CAD build for the part. Positions are in the model's coordinates, mm. Coordinates: 2 decimals unless noted, no trailing zeros. Write each loop counter-clockwise with the first axis right and the second up, starting at its lowest first coordinate (ties: lowest second). Pieces come first, ordered by that corner, then holes. Notation, with made-up numbers: (81.25, 11) -> (102.25, 11) arc R26 ccw to (102.25, 39) -> close; hole circle Ø1 at (46.5, 55.25). An arc over 180 degrees is marked (long way). Answer as CSV lines item,"result".
```python
from build123d import *

# Parameters (mm, degrees)
SKETCH1_W           = 10
SKETCH1_H           = 5
BOSS_EXTRUDE1_DEPTH = 10
SKETCH2_R           = 2.5
CUT_EXTRUDE1_DEPTH  = 171.137369091


with BuildPart() as part:
    # Sketch1 → Boss-Extrude1 (new body)
    with BuildSketch(Plane.XY):
        with Locations((164.769621432, 40.044015335)):
            Rectangle(SKETCH1_W, SKETCH1_H)
    extrude(amount=BOSS_EXTRUDE1_DEPTH)

    # Sketch2 → Cut-Extrude1 (cut, through all)
    with BuildSketch(Plane(origin=(0, 42.544015335, 0), x_dir=(1, 0, 0), z_dir=(0, 1, 0))):
        with Locations(Location((164.769621432, -5, 0), (0, 0, 270))):
            Circle(SKETCH2_R)
        with BuildLine():
            ThreePointArc((169.769621432, -5), (168.305155338, -8.535533906), (164.769621432, -10))
            Line((164.769621432, -10), (169.769621432, -10))
            Line((169.769621432, -10), (169.769621432, -5))
        make_face()
        with BuildLine():
            ThreePointArc((164.769621432, -10), (161.234087527, -8.535533906), (159.769621432, -5))
            Line((159.769621432, -5), (159.769621432, -10))
            Line((159.769621432, -10), (164.769621432, -10))
        make_face()
    extrude(amount=-CUT_EXTRUDE1_DEPTH, mode=Mode.SUBTRACT)


solid = part.part
```
Item 1: Saw through at D-D on x = 161.25. Give the cut face in (y, z), and give its area (3 significant figures).
Answer below:
outline,"(37.54, 0) -> (42.54, 0) -> (42.54, 8.55) -> (37.54, 8.55) -> close"
area,"42.8 mm2"
Item 2: Flat gauge pin, fed straight in: pin 1 (6 mm diameter, centred on x = 164.77, z = 5, fed in from +Y). Where does the tip first touch, or does it go through?
Answer below:
pin 1,"stops at y = 42.54"
Item 3: Saw through at A-A on z = 4. Give the cut face in (x, y).
Answer below:
outline,"(159.77, 37.54) -> (162.48, 37.54) -> (162.48, 42.54) -> (159.77, 42.54) -> close; (167.06, 37.54) -> (169.77, 37.54) -> (169.77, 42.54) -> (167.06, 42.54) -> close"
Item 4: Saw through at B-B on y = 42.1. Give the cut face in (x, z), and give its area (3 significant figures).
Answer below:
outline,"(159.77, 0) -> (169.77, 0) -> (169.77, 5) arc R5 ccw to (159.77, 5) -> close; hole circle Ø5 at (164.77, 5)"
area,"69.6 mm2"
Item 5: Wall check: line 1 (X direction, y = 39.8, z = 5); line 2 (Z direction, x = 164.75, y = 41.1); line 3 (Z direction, x = 167, y = 42). Give the ranges that are in metal, low to high. Write a range as from..to.
Answer below:
line 1,"x = 159.77..162.27, 167.27..169.77"
line 2,"z = 0..2.5, 7.5..10"
line 3,"z = 0..3.87, 6.13..9.47"
Item 6: Two-plate mould, pull along Z, no slides. Class faces 1 (the flat face through (165, 40, 0)), 2 (the flat face through (162, 37.544, 4)), 3 (the cylindrical face through (162.55, 40.08, 6.15)): pulls with the +Z half, pulls with the -Z half, needs draft (parallel to the pull), parting line crosses it, or undercut.
Answer below:
face 1,"pulls with the -Z half"
face 2,"needs draft"
face 3,"undercut"
Item 7: Saw through at C-C on z = 6.25. Give the cut face in (x, y), and give its area (3 significant figures).
Answer below:
outline,"(159.93, 37.54) -> (162.6, 37.54) -> (162.6, 42.54) -> (159.93, 42.54) -> close; (166.93, 37.54) -> (169.61, 37.54) -> (169.61, 42.54) -> (166.93, 42.54) -> close"
area,"26.8 mm2"
